Read the model definition and answer for the solid it produces. Units are mm, in the model's axes. Face numbers are marked on the shaded views. Give positions to 0.01 mm unless a question says otherwise; leave off trailing zeros. Loops run counter-clockwise (first coordinate to the right, second up) from the corner with the lowest first, then second, coordinate; pieces in that order, holes last. Notation, with made-up numbers: (37, 88) -> (91, 88) arc R11 cw to (91, 106) -> close; hole circle Ø8 at (35, -7.5). An arc over 180 degrees is marked (long way). Write each question's results on one line, items separated by ' | '. Start each with the question number.
Item 1: Determine the mould class of the marked faces 1 and 2 for opening direction Y: +Y half, -Y half, draft (parallel to the pull), parting line (faces both ways), or undercut.
Item 2: Section C-C on x = 22.5 is taken. Write down the section's boundary in (y, z).
Item 3: Section B-B on y = 258.5 is taken. Write down the section's boundary in (x, z).
Item 4: Each of these flat-tipped pins is pushed along its axis until it touches: P1, Ø3.5, axis at x = 98, z = 1.5, coming from the -Y side; P2, Ø1.5, axis at x = -78.5, z = 2, coming from the -Y side; P3, Ø1.5, axis at y = 206, z = 1, coming from the +X side; P4, Ø18.5, axis at y = 453.5, z = -13, coming from the +X side. Where does it stop, or does it pass through?
Item 5: Section A-A on x = 117.5 is taken. Write down the section's boundary in (y, z), and give its area (3 significant figures).
Item 6: Find the intervals of material crossed by line 1 (X direction, y = 1.9, z = -15); line 2 (Y direction, x = -13, z = -7.5); line 3 (Y direction, x = 135, z = 1.75), in increasing order.
Item 7: Section D-D on y = 195 is taken. Write down the section's boundary in (x, z).
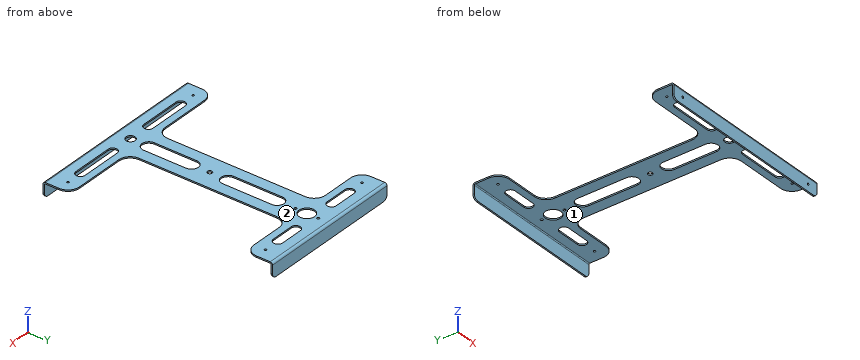
```python
from build123d import *

# Parameters (mm, degrees)
ESQUISSE1_W                             = 400
ESQUISSE1_H                             = 470
BOSS_EXTRU_1_DEPTH                      = 3
T_LE_PLI_E_SUR_AR_TE1_STRIP_W           = 16
T_LE_PLI_E_SUR_AR_TE1_STRIP_H           = 3
T_LE_PLI_E_SUR_AR_TE1_STRIP_CUT_DEPTH   = 400
T_LE_PLI_E_SUR_AR_TE1_STRIP_2_W         = 16
T_LE_PLI_E_SUR_AR_TE1_STRIP_2_H         = 3
T_LE_PLI_E_SUR_AR_TE1_STRIP_CUT_2_DEPTH = 400
T_LE_PLI_E_SUR_AR_TE1_DEPTH             = 400
T_LE_PLI_E_SUR_AR_TE1_BEND_DEPTH        = 400
ENL_V_MAT_EXTRU_1_REACH                 = 513.849
ESQUISSE7_R                             = 5.1
ESQUISSE7_R_2                           = 17
ESQUISSE7_R_3                           = 2.75
ESQUISSE7_R_4                           = 2.25
ENL_V_MAT_EXTRU_6_REACH                 = 513.849
ESQUISSE14_R                            = 10
CONG_10_R                               = 10
CONG_2_R                                = 25
ENL_V_MAT_EXTRU_2_REACH                 = 513.664
ESQUISSE8_R                             = 2.25


# Sheet-metal steps are written as plain solids
with BuildPart() as part:
    # Esquisse1 → Boss.-Extru.1 (new body)
    with BuildSketch(Plane.XY):
        with Locations((0, 235)):
            Rectangle(ESQUISSE1_W, ESQUISSE1_H)
    extrude(amount=BOSS_EXTRU_1_DEPTH)

    # Tôle pliée sur arête1 strip (across the edge) → Tôle pliée sur arête1 strip cut (cut)
    with BuildSketch(Plane(origin=(-200, 470, 0), x_dir=(0, -1, 0), z_dir=(1, 0, 0))):
        with Locations((-3, -1.5)):
            Rectangle(T_LE_PLI_E_SUR_AR_TE1_STRIP_W, T_LE_PLI_E_SUR_AR_TE1_STRIP_H)
    extrude(amount=T_LE_PLI_E_SUR_AR_TE1_STRIP_CUT_DEPTH, mode=Mode.SUBTRACT)

    # Tôle pliée sur arête1 strip 2 (across the edge) → Tôle pliée sur arête1 strip cut 2 (cut)
    with BuildSketch(Plane(origin=(200, 0, 0), x_dir=(0, 1, 0), z_dir=(-1, 0, 0))):
        with Locations((-3, -1.5)):
            Rectangle(T_LE_PLI_E_SUR_AR_TE1_STRIP_2_W, T_LE_PLI_E_SUR_AR_TE1_STRIP_2_H)
    extrude(amount=T_LE_PLI_E_SUR_AR_TE1_STRIP_CUT_2_DEPTH, mode=Mode.SUBTRACT)

    # Tôle pliée sur arête1 section (across the edge) → Tôle pliée sur arête1 (add)
    with BuildSketch(Plane(origin=(-200, 470, 0), x_dir=(0, -1, 0), z_dir=(1, 0, 0))):
        with BuildLine():
            Line((0, 2), (0, 30))
            Line((0, 30), (3, 30))
            Line((3, 30), (3, 2))
            ThreePointArc((3, 2), (3.585786438, 0.585786438), (5, 0))
            Line((5, 0), (5, -3))
            ThreePointArc((5, -3), (1.464466094, -1.535533906), (0, 2))
        make_face()
    extrude(amount=T_LE_PLI_E_SUR_AR_TE1_DEPTH)

    # Tôle pliée sur arête1 section 2 (across the edge) → Tôle pliée sur arête1 bend (add)
    with BuildSketch(Plane(origin=(200, 0, 0), x_dir=(0, 1, 0), z_dir=(-1, 0, 0))):
        with BuildLine():
            Line((0, 2), (0, 30))
            Line((0, 30), (3, 30))
            Line((3, 30), (3, 2))
            ThreePointArc((3, 2), (3.585786438, 0.585786438), (5, 0))
            Line((5, 0), (5, -3))
            ThreePointArc((5, -3), (1.464466094, -1.535533906), (0, 2))
        make_face()
    extrude(amount=T_LE_PLI_E_SUR_AR_TE1_BEND_DEPTH)

    # Esquisse7 → Enlèv. mat.-Extru.1 (cut, up to next)
    with BuildSketch(Plane.XY.offset(3), mode=Mode.PRIVATE) as enl_v_mat_extru_1_sk1:
        with Locations((0, 208)):
            Circle(ESQUISSE7_R)
    enl_v_mat_extru_1_tool1 = extrude(enl_v_mat_extru_1_sk1.sketch, amount=-ENL_V_MAT_EXTRU_1_REACH, mode=Mode.PRIVATE) & part.part
    # Esquisse7 → Enlèv. mat.-Extru.1 (cut, up to next)
    with BuildSketch(Plane.XY.offset(3), mode=Mode.PRIVATE) as enl_v_mat_extru_1_sk2:
        with Locations((0, 420)):
            Circle(ESQUISSE7_R_2)
    enl_v_mat_extru_1_tool2 = extrude(enl_v_mat_extru_1_sk2.sketch, amount=-ENL_V_MAT_EXTRU_1_REACH, mode=Mode.PRIVATE) & part.part
    # Esquisse7 → Enlèv. mat.-Extru.1 (cut, up to next)
    with BuildSketch(Plane.XY.offset(3), mode=Mode.PRIVATE) as enl_v_mat_extru_1_sk3:
        with Locations((0, 445)):
            Circle(ESQUISSE7_R_3)
    enl_v_mat_extru_1_tool3 = extrude(enl_v_mat_extru_1_sk3.sketch, amount=-ENL_V_MAT_EXTRU_1_REACH, mode=Mode.PRIVATE) & part.part
    # Esquisse7 → Enlèv. mat.-Extru.1 (cut, up to next)
    with BuildSketch(Plane.XY.offset(3), mode=Mode.PRIVATE) as enl_v_mat_extru_1_sk4:
        with Locations((0, 395)):
            Circle(ESQUISSE7_R_3)
    enl_v_mat_extru_1_tool4 = extrude(enl_v_mat_extru_1_sk4.sketch, amount=-ENL_V_MAT_EXTRU_1_REACH, mode=Mode.PRIVATE) & part.part
    # Esquisse7 → Enlèv. mat.-Extru.1 (cut, up to next)
    with BuildSketch(Plane.XY.offset(3), mode=Mode.PRIVATE) as enl_v_mat_extru_1_sk5:
        with Locations((-175, 35)):
            Circle(ESQUISSE7_R_4)
    enl_v_mat_extru_1_tool5 = extrude(enl_v_mat_extru_1_sk5.sketch, amount=-ENL_V_MAT_EXTRU_1_REACH, mode=Mode.PRIVATE) & part.part
    # Esquisse7 → Enlèv. mat.-Extru.1 (cut, up to next)
    with BuildSketch(Plane.XY.offset(3), mode=Mode.PRIVATE) as enl_v_mat_extru_1_sk6:
        with Locations((175, 35)):
            Circle(ESQUISSE7_R_4)
    enl_v_mat_extru_1_tool6 = extrude(enl_v_mat_extru_1_sk6.sketch, amount=-ENL_V_MAT_EXTRU_1_REACH, mode=Mode.PRIVATE) & part.part
    # Esquisse7 → Enlèv. mat.-Extru.1 (cut, up to next)
    with BuildSketch(Plane.XY.offset(3), mode=Mode.PRIVATE) as enl_v_mat_extru_1_sk7:
        with Locations((-135, 435)):
            Circle(ESQUISSE7_R_4)
    enl_v_mat_extru_1_tool7 = extrude(enl_v_mat_extru_1_sk7.sketch, amount=-ENL_V_MAT_EXTRU_1_REACH, mode=Mode.PRIVATE) & part.part
    # Esquisse7 → Enlèv. mat.-Extru.1 (cut, up to next)
    with BuildSketch(Plane.XY.offset(3), mode=Mode.PRIVATE) as enl_v_mat_extru_1_sk8:
        with Locations((135, 435)):
            Circle(ESQUISSE7_R_4)
    enl_v_mat_extru_1_tool8 = extrude(enl_v_mat_extru_1_sk8.sketch, amount=-ENL_V_MAT_EXTRU_1_REACH, mode=Mode.PRIVATE) & part.part
    # Esquisse7 → Enlèv. mat.-Extru.1 (cut, up to next)
    with BuildSketch(Plane.XY.offset(3), mode=Mode.PRIVATE) as enl_v_mat_extru_1_sk9:
        Polygon((-200, 60), (-40, 60), (-40, 410), (-160, 410), (-160, 470), (-200, 470), align=None)
    enl_v_mat_extru_1_tool9 = extrude(enl_v_mat_extru_1_sk9.sketch, amount=-ENL_V_MAT_EXTRU_1_REACH, mode=Mode.PRIVATE) & part.part
    # Esquisse7 → Enlèv. mat.-Extru.1 (cut, up to next)
    with BuildSketch(Plane.XY.offset(3), mode=Mode.PRIVATE) as enl_v_mat_extru_1_sk10:
        Polygon((200, 470), (200, 60), (40, 60), (40, 410), (160, 410), (160, 470), align=None)
    enl_v_mat_extru_1_tool10 = extrude(enl_v_mat_extru_1_sk10.sketch, amount=-ENL_V_MAT_EXTRU_1_REACH, mode=Mode.PRIVATE) & part.part
    add(enl_v_mat_extru_1_tool1.solids().sort_by_distance((0, 208, 3))[0], mode=Mode.SUBTRACT)
    add(enl_v_mat_extru_1_tool2.solids().sort_by_distance((0, 420, 3))[0], mode=Mode.SUBTRACT)
    add(enl_v_mat_extru_1_tool3.solids().sort_by_distance((0, 445, 3))[0], mode=Mode.SUBTRACT)
    add(enl_v_mat_extru_1_tool4.solids().sort_by_distance((0, 395, 3))[0], mode=Mode.SUBTRACT)
    add(enl_v_mat_extru_1_tool5.solids().sort_by_distance((-175, 35, 3))[0], mode=Mode.SUBTRACT)
    add(enl_v_mat_extru_1_tool6.solids().sort_by_distance((175, 35, 3))[0], mode=Mode.SUBTRACT)
    add(enl_v_mat_extru_1_tool7.solids().sort_by_distance((-135, 435, 3))[0], mode=Mode.SUBTRACT)
    add(enl_v_mat_extru_1_tool8.solids().sort_by_distance((135, 435, 3))[0], mode=Mode.SUBTRACT)
    add(enl_v_mat_extru_1_tool9.solids().sort_by_distance((-122.465753, 243.424658, 3))[0], mode=Mode.SUBTRACT)
    add(enl_v_mat_extru_1_tool10.solids().sort_by_distance((122.465753, 243.424658, 3))[0], mode=Mode.SUBTRACT)

    # Esquisse14 → Enlèv. mat.-Extru.6 (cut, up to next)
    with BuildSketch(Plane.XY.offset(3), mode=Mode.PRIVATE) as enl_v_mat_extru_6_sk1:
        with Locations((0, 35)):
            Circle(ESQUISSE14_R)
    enl_v_mat_extru_6_tool1 = extrude(enl_v_mat_extru_6_sk1.sketch, amount=-ENL_V_MAT_EXTRU_6_REACH, mode=Mode.PRIVATE) & part.part
    # Esquisse14 → Enlèv. mat.-Extru.6 (cut, up to next)
    with BuildSketch(Plane.XY.offset(3), mode=Mode.PRIVATE) as enl_v_mat_extru_6_sk2:
        with BuildLine():
            Line((-140, 45), (-50, 45))
            ThreePointArc((-50, 45), (-40, 35), (-50, 25))
            Line((-50, 25), (-140, 25))
            ThreePointArc((-140, 25), (-150, 35), (-140, 45))
        make_face()
    enl_v_mat_extru_6_tool2 = extrude(enl_v_mat_extru_6_sk2.sketch, amount=-ENL_V_MAT_EXTRU_6_REACH, mode=Mode.PRIVATE) & part.part
    # Esquisse14 → Enlèv. mat.-Extru.6 (cut, up to next)
    with BuildSketch(Plane.XY.offset(3), mode=Mode.PRIVATE) as enl_v_mat_extru_6_sk3:
        with BuildLine():
            Line((50, 45), (140, 45))
            ThreePointArc((140, 45), (150, 35), (140, 25))
            Line((140, 25), (50, 25))
            ThreePointArc((50, 25), (40, 35), (50, 45))
        make_face()
    enl_v_mat_extru_6_tool3 = extrude(enl_v_mat_extru_6_sk3.sketch, amount=-ENL_V_MAT_EXTRU_6_REACH, mode=Mode.PRIVATE) & part.part
    # Esquisse14 → Enlèv. mat.-Extru.6 (cut, up to next)
    with BuildSketch(Plane.XY.offset(3), mode=Mode.PRIVATE) as enl_v_mat_extru_6_sk4:
        with BuildLine():
            Line((-15, 168), (-15, 75))
            ThreePointArc((-15, 75), (0, 60), (15, 75))
            Line((15, 75), (15, 168))
            ThreePointArc((15, 168), (0, 183), (-15, 168))
        make_face()
    enl_v_mat_extru_6_tool4 = extrude(enl_v_mat_extru_6_sk4.sketch, amount=-ENL_V_MAT_EXTRU_6_REACH, mode=Mode.PRIVATE) & part.part
    # Esquisse14 → Enlèv. mat.-Extru.6 (cut, up to next)
    with BuildSketch(Plane.XY.offset(3), mode=Mode.PRIVATE) as enl_v_mat_extru_6_sk5:
        with BuildLine():
            Line((-15, 355), (-15, 248))
            ThreePointArc((-15, 248), (0, 233), (15, 248))
            Line((15, 248), (15, 355))
            ThreePointArc((15, 355), (0, 370), (-15, 355))
        make_face()
    enl_v_mat_extru_6_tool5 = extrude(enl_v_mat_extru_6_sk5.sketch, amount=-ENL_V_MAT_EXTRU_6_REACH, mode=Mode.PRIVATE) & part.part
    # Esquisse14 → Enlèv. mat.-Extru.6 (cut, up to next)
    with BuildSketch(Plane.XY.offset(3), mode=Mode.PRIVATE) as enl_v_mat_extru_6_sk6:
        with BuildLine():
            Line((100, 445), (50, 445))
            ThreePointArc((50, 445), (40, 435), (50, 425))
            Line((50, 425), (100, 425))
            ThreePointArc((100, 425), (110, 435), (100, 445))
        make_face()
    enl_v_mat_extru_6_tool6 = extrude(enl_v_mat_extru_6_sk6.sketch, amount=-ENL_V_MAT_EXTRU_6_REACH, mode=Mode.PRIVATE) & part.part
    # Esquisse14 → Enlèv. mat.-Extru.6 (cut, up to next)
    with BuildSketch(Plane.XY.offset(3), mode=Mode.PRIVATE) as enl_v_mat_extru_6_sk7:
        with BuildLine():
            Line((-50, 445), (-100, 445))
            ThreePointArc((-100, 445), (-110, 435), (-100, 425))
            Line((-100, 425), (-50, 425))
            ThreePointArc((-50, 425), (-40, 435), (-50, 445))
        make_face()
    enl_v_mat_extru_6_tool7 = extrude(enl_v_mat_extru_6_sk7.sketch, amount=-ENL_V_MAT_EXTRU_6_REACH, mode=Mode.PRIVATE) & part.part
    add(enl_v_mat_extru_6_tool1.solids().sort_by_distance((0, 35, 3))[0], mode=Mode.SUBTRACT)
    add(enl_v_mat_extru_6_tool2.solids().sort_by_distance((-95, 35, 3))[0], mode=Mode.SUBTRACT)
    add(enl_v_mat_extru_6_tool3.solids().sort_by_distance((95, 35, 3))[0], mode=Mode.SUBTRACT)
    add(enl_v_mat_extru_6_tool4.solids().sort_by_distance((0, 121.5, 3))[0], mode=Mode.SUBTRACT)
    add(enl_v_mat_extru_6_tool5.solids().sort_by_distance((0, 301.5, 3))[0], mode=Mode.SUBTRACT)
    add(enl_v_mat_extru_6_tool6.solids().sort_by_distance((75, 435, 3))[0], mode=Mode.SUBTRACT)
    add(enl_v_mat_extru_6_tool7.solids().sort_by_distance((-75, 435, 3))[0], mode=Mode.SUBTRACT)

    # Congé 10
    cong_10_edges = [part.edges().sort_by_distance(p)[0] for p in [
        (160, 468.5, -30),
        (200, 1.5, -30),
        (-200, 1.5, -30),
        (-160, 468.5, -30),
    ]]
    fillet(cong_10_edges, radius=CONG_10_R)

    # Congé2
    cong_2_edges = [part.edges().sort_by_distance(p)[0] for p in [
        (200, 60, 1.5),
        (40, 60, 1.5),
        (40, 410, 1.5),
        (160, 410, 1.5),
        (-200, 60, 1.5),
        (-160, 410, 1.5),
        (-40, 410, 1.5),
        (-40, 60, 1.5),
    ]]
    fillet(cong_2_edges, radius=CONG_2_R)

    # Esquisse8 → Enlèv. mat.-Extru.2 (cut, up to next)
    with BuildSketch(Plane(origin=(0, 0, 0), x_dir=(-1, 0, 0), z_dir=(0, -1, 0)), mode=Mode.PRIVATE) as enl_v_mat_extru_2_sk1:
        with Locations(Location((175, 15, 0), (0, 0, 90))):
            Circle(ESQUISSE8_R)
    enl_v_mat_extru_2_tool1 = extrude(enl_v_mat_extru_2_sk1.sketch, amount=-ENL_V_MAT_EXTRU_2_REACH, mode=Mode.PRIVATE) & part.part
    # Esquisse8 → Enlèv. mat.-Extru.2 (cut, up to next)
    with BuildSketch(Plane(origin=(0, 0, 0), x_dir=(-1, 0, 0), z_dir=(0, -1, 0)), mode=Mode.PRIVATE) as enl_v_mat_extru_2_sk2:
        with Locations(Location((-175, 15, 0), (0, 0, 90))):
            Circle(ESQUISSE8_R)
    enl_v_mat_extru_2_tool2 = extrude(enl_v_mat_extru_2_sk2.sketch, amount=-ENL_V_MAT_EXTRU_2_REACH, mode=Mode.PRIVATE) & part.part
    add(enl_v_mat_extru_2_tool1.solids().sort_by_distance((-175, 0, -15))[0], mode=Mode.SUBTRACT)
    add(enl_v_mat_extru_2_tool2.solids().sort_by_distance((175, 0, -15))[0], mode=Mode.SUBTRACT)


solid = part.part
```
Findings:
1) face 1: undercut | face 2: draft
2) outline: (0, -30) -> (3, -30) -> (3, -2) arc R2 cw to (5, 0) -> (465, 0) arc R2 cw to (467, -2) -> (467, -30) -> (470, -30) -> (470, -2) arc R5 ccw to (465, 3) -> (5, 3) arc R5 ccw to (0, -2) -> close
3) outline: (-40, 0) -> (-15, 0) -> (-15, 3) -> (-40, 3) -> close; (15, 0) -> (40, 0) -> (40, 3) -> (15, 3) -> close
4) P1: y = 0.32 | P2: y = 1.2 | P3: x = 40 | P4: through
5) outline: (0, -30) -> (3, -30) -> (3, -2) arc R2 cw to (5, 0) -> (25, 0) -> (25, 3) -> (5, 3) arc R5 ccw to (0, -2) -> close; (45, 0) -> (60, 0) -> (60, 3) -> (45, 3) -> close; (410, 0) -> (465, 0) arc R2 cw to (467, -2) -> (467, -30) -> (470, -30) -> (470, -2) arc R5 ccw to (465, 3) -> (410, 3) -> close | area: 471 mm2
6) line 1: -200 to -177.25, -172.75 to 172.75, 177.25 to 200 | line 2: 0 to 3, 467 to 470 | line 3: 1.69 to 25, 45 to 60, 410 to 432.75, 437.25 to 468.31
7) outline: (-40, 0) -> (40, 0) -> (40, 3) -> (-40, 3) -> close
